```python
from build123d import *

# Parameters (mm, degrees)
SKETCH011_W   = 130
SKETCH011_H   = 100
PAD005_DEPTH  = 4
SKETCH013_R   = 3.5
HOLE004_DEPTH = 4.001
SKETCH014_R   = 3
HOLE005_DEPTH = 4.001


with BuildPart() as part:
    # Sketch011 → Pad005 (new body)
    with BuildSketch(Plane.XY.offset(76)):
        with Locations((65, -50)):
            Rectangle(SKETCH011_W, SKETCH011_H)
    extrude(amount=PAD005_DEPTH)

    # Sketch013 (on Face6 of Pad005) → Hole004 (cut, through all)
    with BuildSketch(Plane.XY.offset(80)):
        with Locations((110, -80)):
            Circle(SKETCH013_R)
    extrude(amount=-HOLE004_DEPTH, mode=Mode.SUBTRACT)

    # Sketch014 (on Face5 of Hole004) → Hole005 (cut, through all)
    with BuildSketch(Plane.XY.offset(80)):
        with Locations((110, -20)):
            Circle(SKETCH014_R)
    extrude(amount=-HOLE005_DEPTH, mode=Mode.SUBTRACT)


solid = part.part
```
Design review of the part built by this model. Coordinates are the model's own, in mm. Give positions to 0.01 mm unless a question says otherwise; leave off trailing zeros. Loops run counter-clockwise (first coordinate to the right, second up) from the corner with the lowest first, then second, coordinate; pieces in that order, holes last. Notation, with made-up numbers: (75.25, 4) -> (99.25, 4) arc R34 cw to (99.25, 35) -> close; hole circle Ø8 at (74, -8.75). An arc over 180 degrees is marked (long way). One line per item, written item: value.
Q1. We need section B-B on x = 110. Give the boundary of the cut face in (y, z), and give its area (3 significant figures).
Numbers:
outline: (-100, 76) -> (-83.5, 76) -> (-83.5, 80) -> (-100, 80) -> close; (-76.5, 76) -> (-23, 76) -> (-23, 80) -> (-76.5, 80) -> close; (-17, 76) -> (0, 76) -> (0, 80) -> (-17, 80) -> close
area: 348 mm^2
Q2. We need section A-A on y = -80. Give the boundary of the cut face in (x, z).
Numbers:
outline: (0, 76) -> (106.5, 76) -> (106.5, 80) -> (0, 80) -> close; (113.5, 76) -> (130, 76) -> (130, 80) -> (113.5, 80) -> close
Q3. For L1, parallel to Y at x = 110, z = 76.8; L2, parallel to X at y = -18.5, z = 77.25, list the stretches that pass through material, from the lowest coordinate up.
Numbers:
L1: y = -100 to -83.5, -76.5 to -23, -17 to 0
L2: x = 0 to 107.4, 112.6 to 130
Q4. Draft analysis for pull direction X (two halves, no side actions). For faces 1 (the flat face through (130, -51, 78)), 2 (the flat face through (64, 0, 78)), 3 (the cylindrical face through (112.77, -21.15, 78.03)), state which applies: pulls with the +X half, pulls with the -X half, needs draft (parallel to the pull), parting line crosses it, or undercut.
Numbers:
face 1: pulls with the +X half
face 2: needs draft
face 3: undercut
Q5. For pin 1 Ø1.5 at (x, z) = (71, 78) entering from +Y; pin 2 Ø5 at (x, y) = (110, -20) entering from +Z, all flat-tipped, find the tip position at first contact; note any pin that passes through.
Numbers:
pin 1: stops at y = 0
pin 2: passes through
Q6. We need section C-C on y = -20. Give the boundary of the cut face in (x, z), and give its area (3 significant figures).
Numbers:
outline: (0, 76) -> (107, 76) -> (107, 80) -> (0, 80) -> close; (113, 76) -> (130, 76) -> (130, 80) -> (113, 80) -> close
area: 496 mm^2
